Verification items for the finished model (mm, model axes). Round coordinates to 2 decimals unless told otherwise and drop trailing zeros. Order: outer loops, then holes, each group sorted by start corner. A loop starts at its lowest first (then second) coordinate and runs counter-clockwise, first axis right, second up. Notation, with made-up numbers: M 35.5,27.5 L 80.5,27.5 A30 ccw 80.5,56.5 Z; hole C -5,84 d11. An arc over 180 degrees is marked long. Use CSV: the item, a comma, the result in double quotes. Start each with the question number.
Q1. Gauge pin test, flat ends, axial feed: pin 1 Ø2 at (x, z) = (-50.5, -11) entering from +Y; pin 2 Ø6 at (y, z) = (6, 0.5) entering from -X; pin 3 Ø2.5 at (x, y) = (-57.5, 1) entering from +Z. Record the tip position at first contact, or that the pin passes through.
Q2. Scan lines: line 1 (X direction, y = 1.8, z = -20); line 2 (Z direction, x = -45.5, y = 6); line 3 (Y direction, x = -43.75, z = 0). Record each from-to range of solid material in increasing order.
Q3. Sectioned sample at D-D (x = -56). Enter the section's corners in (y, z), and give its area (3 significant figures).
Q4. Sectioned sample at A-A (z = -20). Enter the section's corners in (x, y).
Q5. Sectioned sample at C-C (y = 4). Enter the section's corners in (x, z), and give its area (3 significant figures).
Q6. Sectioned sample at B-B (x = -16). Enter the section's corners in (y, z).
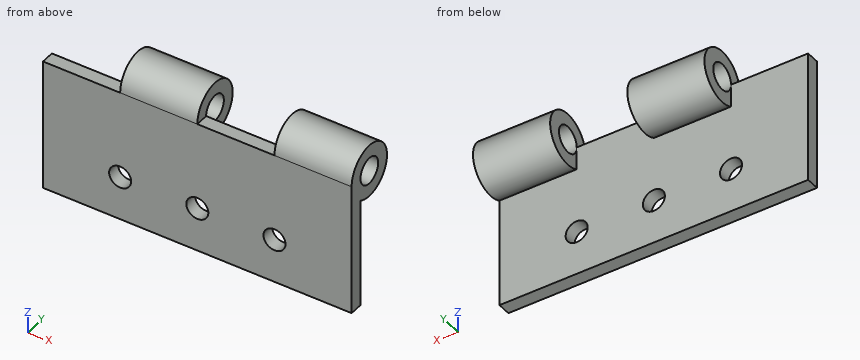
Autodesk Inventor part; units mm, degrees
ref_plane "YZ Plane" through (0, 0, 0) normal (1, 0, 0) x (0, 1, 0)
ref_plane "XZ Plane" through (0, 0, 0) normal (0, 1, 0) x (-1, 0, 0)
ref_plane "XY Plane" through (0, 0, 0) normal (0, 0, 1) x (1, 0, 0)
sketch "Sketch1" plane through (0, 0, 0) normal (0, 1, 0) x (-1, 0, 0)
  line L0 (0, 0) -> (0, -30)
  line L1 (0, -30) -> (70, -30)
  line L2 (70, -30) -> (70, 0)
  line L3 (70, 0) -> (0, 0)
  line L4 (70, -30) -> (70, -20)
  line L5 (70, -20) -> (52.5, -20)
  line L6 (52.5, -20) -> (35, -20)
  line L7 (35, -20) -> (17.5, -20)
  circle A0 centre (52.5, -20) radius 2.5
  circle A1 centre (35, -20) radius 2.5
  circle A2 centre (17.5, -20) radius 2.5
  dimension "d0" = 30
  dimension "d1" = 70
  dimension "d2" = 10
  dimension "d3" = 17.5
  dimension "d4" = 17.5
  dimension "d5" = 17.5
  dimension "d6" = 5
  dimension "d7" = 5
  dimension "d8" = 5
extrude "Extrusion1" add sketch "Sketch1" along normal blind 3
sketch "Sketch2" plane through (0, 0, 0) normal (1, 0, 0) x (0, 0, -1)
  line L0 (0, 3) -> (30, 3)
  circle A0 centre (0, 6) radius 3
  line L1 (0, 0) -> (0, 3)
  circle A1 centre (0, 6) radius 6
extrude "Extrusion2" add sketch "Sketch2" against normal blind 70 contours L1 A1 L0 | A0 | L0 A1 L1
sketch "Sketch3" plane through (0, 0, -30) normal (1, 0, 0) x (0, 0, -1)
  line L0 (-30, 0) -> (0, 0)
  line L1 (-30, 0) -> (-30, 6)
  circle A0 centre (-30, 6) radius 3
  dimension "d14" = 6
  dimension "d15" = 6
extrude "Extrusion3" cut sketch "Sketch3" against normal blind 70
sketch "Sketch4" plane through (0, 0, -30) normal (0, 0, -1) x (-1, 0, 0)
  line L0 (0, 0) -> (70, 0)
  line L1 (0, 0) -> (0, 3)
  line L2 (0, 3) -> (70, 3)
  line L3 (0, 3) -> (17.5, 3)
  line L4 (17.5, 3) -> (35, 3)
  line L5 (35, 3) -> (52.5, 3)
  line L6 (52.5, 3) -> (70, 3)
  line L7 (70, 0) -> (70, 12)
  line L8 (70, 3) -> (70, 12)
  line L9 (70, 12) -> (52.5, 12)
  line L10 (0, 12) -> (70, 12)
  line L11 (52.5, 3) -> (52.5, 12)
  line L12 (17.5, 3) -> (17.5, 12)
  line L13 (17.5, 12) -> (35, 12)
  line L14 (35, 12) -> (35, 3)
  dimension "d18" = 17.5
  dimension "d19" = 17.5
  dimension "d20" = 17.5
extrude "Extrusion4" cut sketch "Sketch4" against normal blind 70 contours L2 L11 L9 L7 | L12 L10 L14 L2
sketch "Sketch5" plane through (0, 3, 0) normal (0, 1, 0) x (1, 0, 0)
  line L0 (-17.5, -5.1962) -> (-35, -5.1962)
  line L1 (-35, 6) -> (-35, -6)
  line L2 (-35, 0) -> (-35, -5.1962)
  line L3 (-35, -5.1962) -> (-17.5, -5.1962)
  line L4 (-17.5, -5.1962) -> (-17.5, 0)
  line L5 (-17.5, 0) -> (-35, 0)
  line L6 (-35, 5.1962) -> (-35, 0)
  line L7 (-35, 0) -> (-35, -5.1962)
  line L8 (-52.5, -5.1962) -> (-70, -5.1962)
  line L9 (-52.5, -5.1962) -> (-70, -5.1962)
  line L10 (-70, 0) -> (-70, -5.1962)
  line L11 (-70, -5.1962) -> (-70, 0)
  line L12 (-70, 0) -> (-52.5, 0)
  line L13 (-70, 0) -> (0, 0)
  line L14 (-52.5, 0) -> (-52.5, -5.1962)
  line L15 (-52.5, 5.1962) -> (-52.5, 0)
  line L16 (-52.5, -5.1962) -> (-52.5, 0)
  dimension "d24" = 17.5
extrude "Extrusion5" cut sketch "Sketch5" against normal blind 70
properties part number "Dobradiça"
Verdict:
1,pin 1,"stops at y = 3"
1,pin 2,"stops at x = -52.5"
1,pin 3,"stops at z = 0"
2,line 1,"x = -70 to -55, -50 to -37.5, -32.5 to -20, -15 to 0"
2,line 2,"z = -6 to -3, 3 to 6"
2,line 3,"y = 0 to 3, 9 to 12"
3,outline,"M 0,-30 L 3,-30 L 3,0 L 0,0 Z"
3,area,"90.0 mm²"
4,outline,"M -70,0 L -55,0 L -55,3 L -70,3 Z; M -50,0 L -37.5,0 L -37.5,3 L -50,3 Z; M -32.5,0 L -20,0 L -20,3 L -32.5,3 Z; M -15,0 L 0,0 L 0,3 L -15,3 Z"
5,outline,"M -52.5,-5.66 L -35,-5.66 L -35,-2.24 L -52.5,-2.24 Z; M -52.5,2.24 L -35,2.24 L -35,5.66 L -52.5,5.66 Z; M -17.5,-5.66 L 0,-5.66 L 0,-2.24 L -17.5,-2.24 Z; M -17.5,2.24 L 0,2.24 L 0,5.66 L -17.5,5.66 Z"
5,area,"239 mm²"
6,outline,"M 0,-30 L 3,-30 L 3,-22 L 0,-22 Z; M 0,-18 L 3,-18 L 3,-5.2 A6 ccw long 0,0 Z; hole C 6,0 d6"
